```python
from build123d import *

# Parameters (mm, degrees)
ESBO_O2_W                = 80
ESBO_O2_H                = 80
RESSALTO_EXTRUS_O2_DEPTH = 22.225
ESBO_O10_R               = 4
ESBO_O10_R_2             = 3
CORTE_EXTRUS_O5_DEPTH    = 30
ESBO_O12_R               = 10
CORTE_EXTRUS_O7_DEPTH    = 81


with BuildPart() as part:
    # Esboço2 → Ressalto-extrusão2 (new body, symmetric)
    with BuildSketch(Plane.XY):
        Rectangle(ESBO_O2_W, ESBO_O2_H)
    extrude(amount=RESSALTO_EXTRUS_O2_DEPTH, both=True)

    # Esboço10 → Corte-extrusão5 (cut)
    with BuildSketch(Plane(origin=(0, 40, 0), x_dir=(1, 0, 0), z_dir=(0, 1, 0))):
        with Locations((30, -12.225)):
            Circle(ESBO_O10_R)
        with Locations((30, 12.225)):
            Circle(ESBO_O10_R)
        with Locations((-30, -12.225)):
            Circle(ESBO_O10_R)
        with Locations((-30, 12.225)):
            Circle(ESBO_O10_R)
        with Locations((15, 0)):
            Circle(ESBO_O10_R_2)
        with Locations((-15, 0)):
            Circle(ESBO_O10_R_2)
    extrude(amount=-CORTE_EXTRUS_O5_DEPTH, mode=Mode.SUBTRACT)

    # Esboço12 → Corte-extrusão7 (cut, through all)
    with BuildSketch(Plane(origin=(40, 0, 0), x_dir=(0, 0, -1), z_dir=(1, 0, 0))):
        with Locations((0, -15.9)):
            Circle(ESBO_O12_R)
    extrude(amount=-CORTE_EXTRUS_O7_DEPTH, mode=Mode.SUBTRACT)


solid = part.part
```
Source: CAD feature listing. Evaluate the final solid. Frame: model axes, mm. A direction names the side the tool comes from. Coordinates: 2 decimals unless noted, no trailing zeros. Loops run counter-clockwise (first coordinate to the right, second up) from the corner with the lowest first, then second, coordinate; pieces in that order, holes last. Notation, with made-up numbers: M 6,0 L 41,0 A32 cw 41,39 Z; hole C 7,79 d9. An arc over 180 degrees is marked long. Put each result on its own line as item: value. Start each with the question number.
1) Cut plane D-D on x = 30. Return the cut outline in (y, z) (3 decimals).
2) Pull-direction query (X, two-part tool) for faces 3 (the face through (-1, -40, 0)), 4 (the face through (29.13, 25.21, -8.32)), 5 (the face through (-40, -1, 0)); classes: pulls with the +X half, pulls with the -X half, needs draft (parallel to the pull), parting line crosses it, or undercut.
3) Cut plane C-C on z = 0. Return the cut outline in (x, y), then the cut area to 3 significant figures.
4) Contact query for a flat-ended pin moving along its axis: pin 1 Ø4 at (x, z) = (31.5, -11) entering from +Y. Output: stop coordinate, or through.
5) Cut plane B-B on x = -15. Return the cut outline in (y, z) (3 decimals).
6) Cut plane A-A on y = -15.9. Return the cut outline in (x, z) (3 decimals), then the cut area to 3 significant figures.
7) Ray query, L1, parallel to Z at x = -30, y = 24.75 (3 decimals); L2, parallel to X at y = 17.5, z = 0; L3, parallel to Z at x = 15, y = 33 (3 decimals). Return the intervals inside material, ascending. Write a range as from..to.
8) Reachability of faces 1 (the face through (-18, 25, 0)), 2 (the face through (-1, 40, 0)) from +Z, -Z, +X, -X, +Y, -Y: full face, straight path, thin tool, end or side. Return the list, or none.
The answers:
1. outline: M -40,-22.225 L 40,-22.225 L 40,-16.225 L 10,-16.225 L 10,-8.225 L 40,-8.225 L 40,8.225 L 10,8.225 L 10,16.225 L 40,16.225 L 40,22.225 L -40,22.225 Z; hole C -15.9,0 d20
2. face 3: needs draft
2. face 4: undercut
2. face 5: pulls with the -X half
3. outline: M -40,-40 L 40,-40 L 40,-25.9 L -40,-25.9 Z; M -40,-5.9 L 40,-5.9 L 40,40 L 18,40 L 18,10 L 12,10 L 12,40 L -12,40 L -12,10 L -18,10 L -18,40 L -40,40 Z
3. area: 4,440 mm²
4. pin 1: stops at y = 10
5. outline: M -40,-22.225 L 40,-22.225 L 40,-3 L 10,-3 L 10,3 L 40,3 L 40,22.225 L -40,22.225 Z; hole C -15.9,0 d20
6. outline: M -40,-22.225 L 40,-22.225 L 40,-10 L -40,-10 Z; M -40,10 L 40,10 L 40,22.225 L -40,22.225 Z
6. area: 1,960 mm²
7. L1: z = -22.225..-16.225, -8.225..8.225, 16.225..22.225
7. L2: x = -40..-18, -12..12, 18..40
7. L3: z = -22.225..-3, 3..22.225
8. face 1: +Y
8. face 2: +Z, -Z, +X, -X, +Y
